Could you check a few things on this drawing? It's one solid part, dimensions in mm from its lowest x, y, z. A direction names the side the tool comes from. Round coordinates to 2 decimals unless told otherwise and drop trailing zeros. Loops run counter-clockwise (first coordinate to the right, second up) from the corner with the lowest first, then second, coordinate; pieces in that order, holes last. Notation, with made-up numbers: M 69.25,29 L 94.25,29 A14 ccw 94.25,36 Z; hole C 43.25,87.5 d8. An arc over 180 degrees is marked long. Return JSON: item names as keys, results as strings.
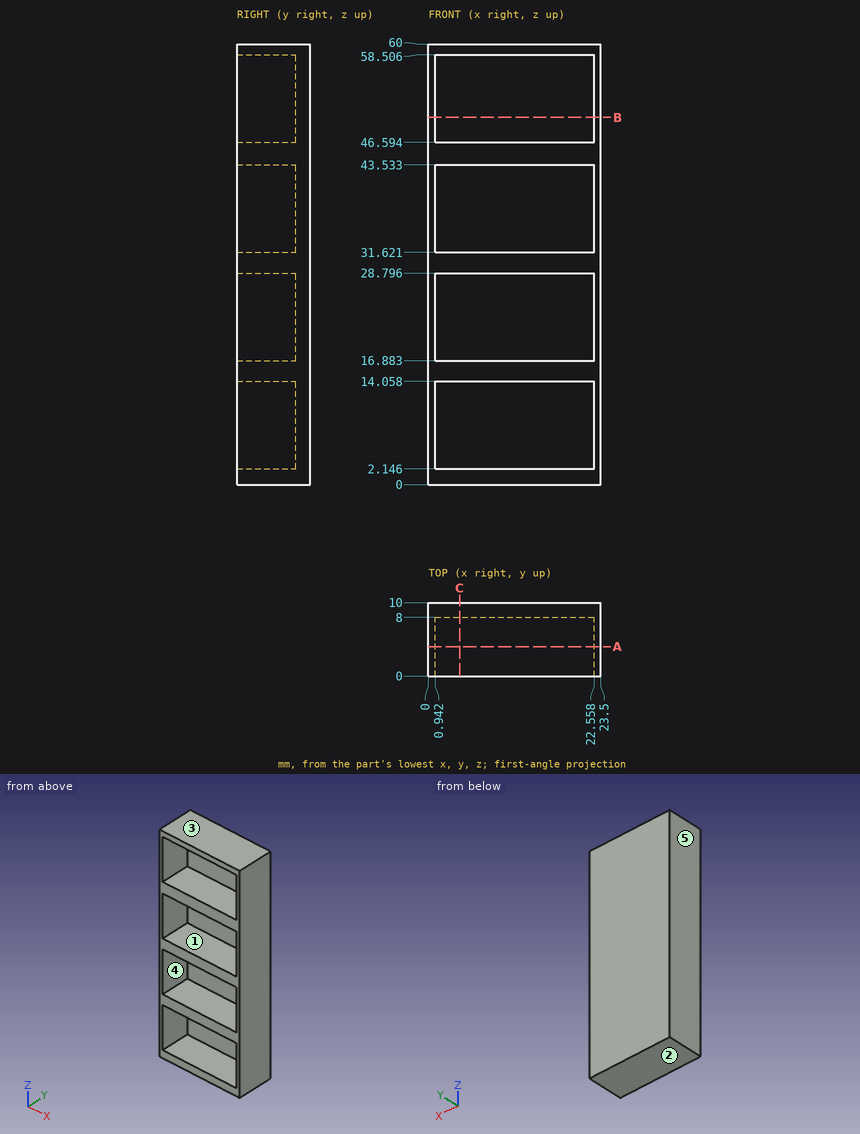
Q1. Suppose I cut it at A-A, the plane y = 4. Please give me the cut outline in (x, z) (1 decimal), plus the area to 3 significant figures.
Results:
{"outline": "M 0,0 L 23.5,0 L 23.5,60 L 0,60 Z; hole M 0.9,2.1 L 22.6,2.1 L 22.6,14.1 L 0.9,14.1 Z; hole M 0.9,16.9 L 22.6,16.9 L 22.6,28.8 L 0.9,28.8 Z; hole M 0.9,31.6 L 22.6,31.6 L 22.6,43.5 L 0.9,43.5 Z; hole M 0.9,46.6 L 22.6,46.6 L 22.6,58.5 L 0.9,58.5 Z", "area": "380 mm2"}
Q2. Thinking about a two-plate mould opening in Z: for the marked faces 3, 4 and 5, which applies, pulls with the +Z half, pulls with the -Z half, needs draft (parallel to the pull), parting line crosses it, or undercut?
Results:
{"face 3": "pulls with the +Z half", "face 4": "undercut", "face 5": "needs draft"}
Q3. Suppose I cut it at C-C, the plane x = 4.25. Please give me the cut outline in (y, z) (1 decimal), plus the area to 3 significant figures.
Results:
{"outline": "M 0,0 L 10,0 L 10,60 L 0,60 L 0,58.5 L 8,58.5 L 8,46.6 L 0,46.6 L 0,43.5 L 8,43.5 L 8,31.6 L 0,31.6 L 0,28.8 L 8,28.8 L 8,16.9 L 0,16.9 L 0,14.1 L 8,14.1 L 8,2.1 L 0,2.1 Z", "area": "219 mm2"}
Q4. Suppose I cut it at B-B, the plane z = 50. Please give me the cut outline in (x, y).
Results:
{"outline": "M 0,0 L 0.94,0 L 0.94,8 L 22.56,8 L 22.56,0 L 23.5,0 L 23.5,10 L 0,10 Z"}
Q5. On a 3-axis mill with a long thin cutter (end or side, diameter ignored), from which of +Z, -Z, +X, -X, +Y, -Y can I reach the whole of each face in a straight line? I mean the marked faces 1 and 2. Say none if no direction works.
Results:
{"face 1": "-Y", "face 2": "-Z, +X, -X, +Y, -Y"}
Q6. If I drill on line 1 along Z through (x, y) = (7, 3) (1 decimal); line 2 along X through (y, z) = (5.5, 54.5); line 3 along Y through (x, z) = (11.5, 19.5), over which ranges is the centre line in solid material (lowest first)?
Results:
{"line 1": "z = 0 to 2.1, 14.1 to 16.9, 28.8 to 31.6, 43.5 to 46.6, 58.5 to 60", "line 2": "x = 0 to 0.94, 22.56 to 23.5", "line 3": "y = 8 to 10"}
Q7. I'm going to push a flat-ended pin straight in: pin 1 Ø6 at (x, z) = (12.5, 10) entering from -Y. Where does the tip first touch, or does it pass through?
Results:
{"pin 1": "stops at y = 8"}
